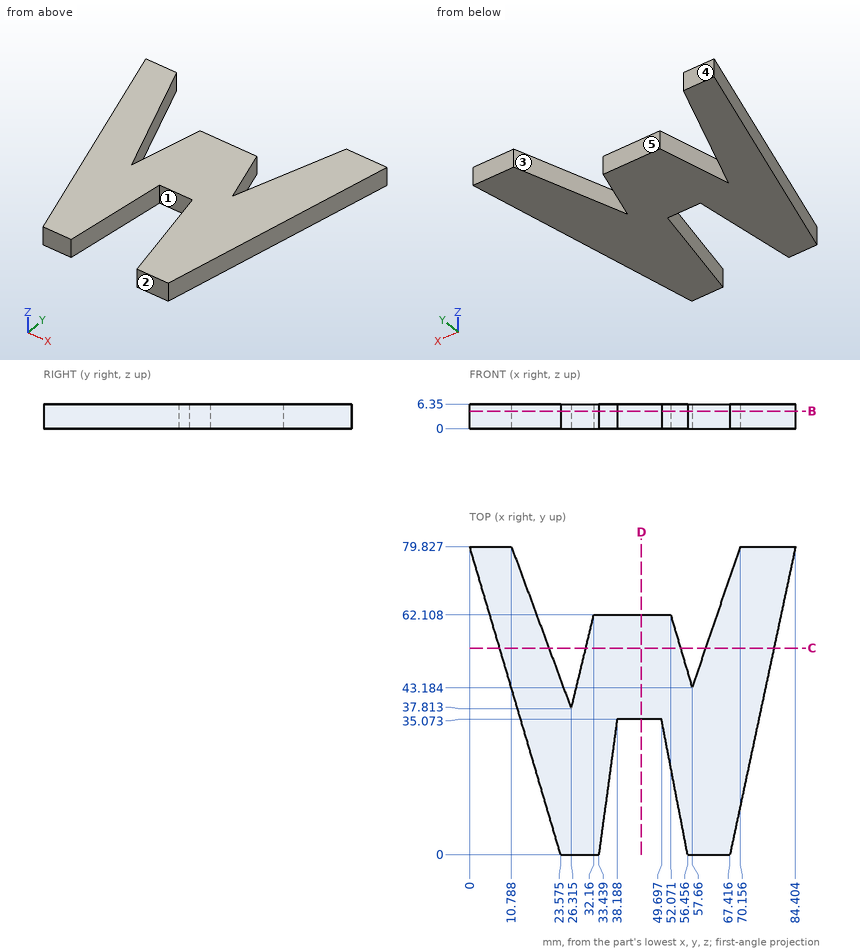
Could you check a few things on this drawing? It's one solid part, dimensions in mm from its lowest x, y, z. A direction names the side the tool comes from. Give positions to 0.01 mm unless a question says otherwise; leave off trailing zeros. Loops run counter-clockwise (first coordinate to the right, second up) from the corner with the lowest first, then second, coordinate; pieces in that order, holes last. Notation, with made-up numbers: M 19,-36 L 43,-36 A22 cw 43,-21 Z; hole C 1.25,-15 d5. An arc over 180 degrees is marked long. One line per question, with ' | ' between items. Start each with the question number.
Q1. If we mould it in two halves opening along X, with no side actions, what happens to the marked faces 4 and 5? For each: +X half, -X half, draft (parallel to the pull), parting line (faces both ways), or undercut.
Q2. If we section it at B-B (z = 4.5): Please give me the cut outline in (x, y) (1 decimal).
Q3. If I drill on line 1 (X direction, y = 44, z = 5.5) (1 decimal); line 2 (X direction, y = 27, z = 5.5) (1 decimal); line 3 (X direction, y = 76.5, z = 4.75) (1 decimal), over which ranges is the centre line in solid material (lowest first)? Write a range as from..to.
Q4. For the marked faces 1, 2 and 3, which set-ups out of +Z, -Z, +X, -X, +Y, -Y let a thin tool reach every point of the face, with its end or its side?
Q5. For pin 1 Ø2 at (y, z) = (11, 1.5) entering from -X; pin 2 Ø4 at (x, y) = (38, 25) entering from -Z; pin 3 Ø1.9 at (x, z) = (43.5, 2) entering from +Y; pin 4 Ø3 at (y, z) = (53.5, 5) entering from +X, each with a flat end and sliding along its axis, tell me the tip position at first contact or that it passes through.
Q6. If we section it at C-C (y = 53.5): State how many separate pieces and enclosed holes the cut face has.
Q7. If we section it at D-D (x = 44.5): Please give me the cut outline in (y, z).
Computed:
1) face 4: draft | face 5: undercut
2) outline: M 0,79.8 L 23.6,0 L 33.4,0 L 38.2,35.1 L 49.7,35.1 L 56.5,0 L 67.4,0 L 84.4,79.8 L 70.2,79.8 L 57.7,43.2 L 52.1,62.1 L 32.2,62.1 L 26.3,37.8 L 10.8,79.8 Z
3) line 1: x = 10.6..24, 27.8..57.4, 57.9..76.8 | line 2: x = 15.6..37.1, 51.3..73.2 | line 3: x = 1..12, 69..83.7
4) face 1: +Z, -Z, -Y | face 2: +Z, -Z, +X, -X, -Y | face 3: +Z, -Z, +Y
5) pin 1: stops at x = 20.03 | pin 2: stops at z = 0 | pin 3: stops at y = 62.11 | pin 4: stops at x = 79.12
6) separate pieces: 3 | enclosed holes: 0
7) outline: M 35.07,0 L 62.11,0 L 62.11,6.35 L 35.07,6.35 Z
